from build123d import *

# Parameters (mm, degrees)
SKETCH1_R           = 2.54
BOSS_EXTRUDE1_DEPTH = 3.175


with BuildPart() as part:
    # Sketch1 → Boss-Extrude1 (new body)
    with BuildSketch(Plane.XY):
        with BuildLine():
            Line((0, 27.813), (0, 26.543))
            ThreePointArc((0, 26.543), (-7.215038926, 21.131730585), (-4.040445833, 12.690132272))
            ThreePointArc((-4.040445833, 12.690132272), (-0.676998183, 3.691361084), (-9.855894217, 0.856130829))
            ThreePointArc((-9.855894217, 0.856130829), (-11.652031758, 18.448211646), (0, 31.75))
            Line((0, 31.75), (0, 30.48))
            ThreePointArc((0, 30.48), (-1.3335, 29.1465), (0, 27.813))
        make_face()
        with Locations((-6.604, 6.604)):
            Circle(SKETCH1_R, mode=Mode.SUBTRACT)
    extrude(amount=BOSS_EXTRUDE1_DEPTH)


solid = part.part
For this review, take the finished solid that the model builds, in its own axes (mm). Round coordinates to 2 decimals unless told otherwise and drop trailing zeros. Loops run counter-clockwise (first coordinate to the right, second up) from the corner with the lowest first, then second, coordinate; pieces in that order, holes last. Notation, with made-up numbers: (-9.5, 7.25) - (40.5, 7.25) arc R17 cw to (40.5, 39.25) - close; hole circle Ø10 at (-27, -9.75). An arc over 180 degrees is marked (long way). Use one line per item in the form item = value.
1) Wall thickness on probe 1 along Y at (x, z) = (-6, 0.95); probe 2 along Y at (x, z) = (-4.5, 2.95); probe 3 along Y at (x, z) = (-8, 0.95): over which ranges is each line inside the solid? List them lowest first.
Solutions:
probe_1 = 0.03 to 4.14, 9.07 to 14.5, 23.55 to 27.59
probe_2 = 0.34 to 5.18, 8.03 to 13.01, 25.05 to 28.92
probe_3 = 0.15 to 4.48, 8.73 to 25.36
2) We need section A-A on x = -2.25. Write out the cut boundary in (y, z) (3 decimals), then the cut area to 3 significant figures.
Solutions:
outline = (1.639, 0) - (11.569, 0) - (11.569, 3.175) - (1.639, 3.175) - close; (26.198, 0) - (30.525, 0) - (30.525, 3.175) - (26.198, 3.175) - close
area = 45.3 mm2
3) We need section B-B on y = 4.5. Write out the cut boundary in (x, z) (3 decimals).
Solutions:
outline = (-11.492, 0) - (-8.027, 0) - (-8.027, 3.175) - (-11.492, 3.175) - close; (-5.181, 0) - (-0.344, 0) - (-0.344, 3.175) - (-5.181, 3.175) - close
4) We need section D-D on z = 1.9. Write out the cut boundary in (x, y), then the cut area to 3 significant figures.
Solutions:
outline = (-9.86, 0.86) arc R6.6 ccw (long way) to (-4.04, 12.69) arc R7.52 cw to (0, 26.54) - (0, 27.81) arc R1.33 cw to (0, 30.48) - (0, 31.75) arc R22.15 ccw to start; hole circle Ø5.08 at (-6.6, 6.6)
area = 193 mm2
5) We need section C-C on x = -6. Write out the cut boundary in (y, z) (3 decimals), then the cut area to 3 significant figures.
Solutions:
outline = (0.028, 0) - (4.137, 0) - (4.137, 3.175) - (0.028, 3.175) - close; (9.071, 0) - (14.501, 0) - (14.501, 3.175) - (9.071, 3.175) - close; (23.553, 0) - (27.588, 0) - (27.588, 3.175) - (23.553, 3.175) - close
area = 43.1 mm2
6) Clearance check with flat-ended pins moving along their axes: P1, Ø1.5, axis at x = -10, z = 0.5, coming from the +Y side; P2, Ø1, axis at y = 4, z = 3, coming from the -X side. State where each tip first meets the part, or that it passes through.
Solutions:
P1 = 23.59
P2 = -11.49
7) Mouldability with a two-part tool opening along Y and no side actions: class faces 1 (the face through (-11.728, 18.205, 1.565)), 2 (the face through (-6, 13, 0)), 3 (the face through (-0.61, 3.83, 1.57)) as pulls with the +Y half, pulls with the -Y half, needs draft (parallel to the pull), parting line crosses it, or undercut.
Solutions:
face_1 = parting line crosses it
face_2 = needs draft
face_3 = undercut
